Solid Edge part; units mm, degrees
sketch "Sketch1" plane through (0, 0, 0) normal (0, -1, 0) x (1, 0, 0)
  arc A0 (-24.229, 30.7837) -> (-8.3881, -38.2664) centre (0, 0) cw
  line L0 (-8.3881, -38.2664) -> (-78.0589, -22.9945)
  arc A1 (-85.6745, -24.3941) -> (-78.0589, -22.9945) centre (-80.2, -32.7626) cw
  line L1 (-105.5582, -37.4017) -> (-85.6745, -24.3941)
  arc A2 (-105.5582, -37.4017) -> (-111.3055, -12.3495) centre (-113.0582, -25.937) cw
  line L2 (-111.3055, -12.3495) -> (-87.7403, -15.3893)
  arc A3 (-87.7403, -15.3893) -> (-80.2761, -13.3295) centre (-86.4609, -5.4715) ccw
  line L3 (-24.229, 30.7837) -> (-80.2761, -13.3295)
  arc A4 (-22.5591, 28.662) -> (-7.81, -35.6291) centre (0, 0) cw
  line L4 (-7.81, -35.6291) -> (-77.4807, -20.3571)
  arc A5 (-77.4807, -20.3571) -> (-87.1526, -22.1347) centre (-80.2, -32.7626) ccw
  line L5 (-87.1526, -22.1347) -> (-107.0363, -35.1422)
  arc A6 (-107.0363, -35.1422) -> (-111.6509, -15.0274) centre (-113.0582, -25.937) cw
  line L6 (-88.0857, -18.0672) -> (-111.6509, -15.0274)
  arc A7 (-78.6062, -15.4512) -> (-88.0857, -18.0672) centre (-86.4609, -5.4715) cw
  line L7 (-22.5591, 28.662) -> (-78.6062, -15.4512)
extrude "Protrusion1" add sketch "Sketch1" against normal blind 10
properties part number "1976-1100-C01" material "Poliuretano"
The model under review builds one solid part; all positions refer to its coordinate system, in mm. A direction names the side the tool comes from. Give positions to 0.01 mm unless a question says otherwise; leave off trailing zeros. Order: outer loops, then holes, each group sorted by start corner. A loop starts at its lowest first (then second) coordinate and runs counter-clockwise, first axis right, second up. Notation, with made-up numbers: (61.5, 11.25) - (85.5, 11.25) arc R25 cw to (85.5, 32.25) - close; hole circle Ø2 at (-0.5, 43.5). An arc over 180 degrees is marked (long way). Use CSV: the item, a comma, the result in double quotes. Start each with the question number.
Q1. To check wall thickness, follow line 1 along Z through (x, y) = (-2.5, 7.25); line 2 along X through (y, z) = (6, 0) (3 decimals); line 3 along Z through (x, y) = (-20, 4.75). State the ranges of each line that lie inside material, in increasing order. Write a range as [from, to].
Q2. Tool access review of faces 5 (the flat face through (-42.736, 4.93, -30.737)), 6 (the flat face through (-99.7, 4.93, -16.57)), 7 (the cylindrical face through (-83.854, 4.93, -15.126)): name each direction out of +Z, -Z, +X, -X, +Y, -Y from which nothing blocks a thin tool from reaching the whole face with its end or side.
Q3. We need section A-A, the plane x = 0. Write out the cut boundary in (y, z) (3 decimals).
Q4. Clearance check with flat-ended pins moving along their axes: pin 1 Ø5 at (x, y) = (-60, 8.5) entering from +Z; pin 2 Ø5 at (x, y) = (-87, 1.5) entering from -Z; pin 3 Ø2 at (y, z) = (3.5, -29) entering from -X. State where each tip first meets the part, or that it passes through.
Q5. We need section C-C, the plane z = 5. Write out the cut boundary in (x, y).
Q6. The part is to be moulded in two halves that separate along Z. For faces 1 (the flat face through (-95.76, 4.93, -30.99)), 2 (the flat face through (-37, 0, -30)), 3 (the cylindrical face through (-83.151, 4.93, -17.733)), 4 (the flat face through (-99.688, 4.93, -13.848)), say which applies: +Z half, -Z half, draft (parallel to the pull), parting line (faces both ways), or undercut.
Outcome:
1,line 1,"z = [-39.1, -36.39], [36.39, 39.1]"
1,line 2,"x = [-63.341, -58.975], [36.475, 39.175]"
1,line 3,"z = [-35.72, -32.96], [30.5, 33.69]"
2,face 5,"-Z, +Y, -Y"
2,face 6,"+Y, -Y"
2,face 7,"+Z, +Y, -Y"
3,outline,"(0, -39.175) - (10, -39.175) - (10, -36.475) - (0, -36.475) - close; (0, 36.475) - (10, 36.475) - (10, 39.175) - (0, 39.175) - close"
4,pin 1,"stops at z = 4.6"
4,pin 2,"stops at z = -26.9"
4,pin 3,"stops at x = -126.6"
5,outline,"(-56.99, 0) - (-52.62, 0) - (-52.62, 10) - (-56.99, 10) - close; (36.13, 0) - (38.85, 0) - (38.85, 10) - (36.13, 10) - close"
6,face 1,"-Z half"
6,face 2,"draft"
6,face 3,"undercut"
6,face 4,"+Z half"
